Read the model definition and answer for the solid it produces. Units are mm, in the model's axes. Round coordinates to 2 decimals unless told otherwise and drop trailing zeros. Write each loop counter-clockwise with the first axis right and the second up, starting at its lowest first coordinate (ties: lowest second). Pieces come first, ordered by that corner, then holes. Notation, with made-up numbers: (3, -11) - (45, -11) arc R23 ccw to (45, 27) - close; hole circle Ø4 at (56, -14). An arc over 180 degrees is marked (long way). Answer as CSV lines item,"result". Start each with the question number.
1) Find section A-A on x = 0. Determine the outline of the cut face in (y, z) (3 decimals), then the cut area to 3 significant figures.
2) Consider line 1 along Y through (x, z) = (0, -0.4); line 2 along Y through (x, z) = (-0.5, -3); line 3 along X through (y, z) = (15, -2.9) (3 decimals). Determine where each line is inside the solid, lowest interval first.
3) Find section D-D on z = -4. Determine the outline of the cut face in (x, y) (3 decimals), then the cut area to 3 significant figures.
4) Find section C-C on y = 26. Determine the outline of the cut face in (x, z).
5) Each of these flat-tipped pins is pushed along its axis until it touches: pin 1 (2 mm diameter, centred on x = -1.5, y = 15.5, fed in from +Z); pin 2 (2 mm diameter, centred on x = 4.5, y = 54, fed in from +Z); pin 3 (1 mm diameter, centred on y = 36.5, z = -1.5, fed in from -X). Where does it stop, or does it pass through?
6) Find section B-B on y = 45. Determine the outline of the cut face in (x, z) (3 decimals).
from build123d import *

# Parameters (mm, degrees)
BOSS_EXTRUDE1_DEPTH                       = 60
TAPPED_HOLE_FOR_M2_5X0_45_HELICOIL1_D     = 2.55
TAPPED_HOLE_FOR_M2_5X0_45_HELICOIL1_DEPTH = 4
TAPPED_HOLE_FOR_M2_5X0_45_HELICOIL1_TIP   = 0.766097289
F_2_0MM_DOWEL_HOLE1_D                     = 2
F_2_0MM_DOWEL_HOLE1_DEPTH                 = 6.45
F_2_0MM_DOWEL_HOLE1_TIP                   = 0.600860619


with BuildPart() as part:
    # Sketch1 → Boss-Extrude1 (new body)
    with BuildSketch(Plane(origin=(0, 0, 0), x_dir=(1, 0, 0), z_dir=(0, 1, 0))):
        with BuildLine():
            Line((-0.716915426, 0), (0.716915426, 0))
            ThreePointArc((0.716915426, 0), (3.210792252, 3.53742677), (7, 5.629008568))
            Line((7, 5.629008568), (7, 6))
            Line((7, 6), (-7, 6))
            Line((-7, 6), (-7, 5.629008568))
            ThreePointArc((-7, 5.629008568), (-3.210792252, 3.53742677), (-0.716915426, 0))
        make_face()
    extrude(amount=BOSS_EXTRUDE1_DEPTH)

    # Tapped Hole for M2.5x0.45 Helicoil1
    with Locations(Plane(origin=(0, 45, -6), x_dir=(-1, 0, 0), z_dir=(0, 0, -1))):
        with Locations((0, 0), (0, -30)):
            Hole(TAPPED_HOLE_FOR_M2_5X0_45_HELICOIL1_D / 2, depth=TAPPED_HOLE_FOR_M2_5X0_45_HELICOIL1_DEPTH)
            with Locations((0, 0, -(TAPPED_HOLE_FOR_M2_5X0_45_HELICOIL1_DEPTH + TAPPED_HOLE_FOR_M2_5X0_45_HELICOIL1_TIP / 2))):  # 118° drill point
                Cone(0, TAPPED_HOLE_FOR_M2_5X0_45_HELICOIL1_D / 2, TAPPED_HOLE_FOR_M2_5X0_45_HELICOIL1_TIP, mode=Mode.SUBTRACT)

    # Ø2.0mm Dowel Hole1
    with Locations(Plane(origin=(0, 45, -6), x_dir=(-1, 0, 0), z_dir=(0, 0, -1))):
        with Locations((0, 0), (0, -30)):
            Hole(F_2_0MM_DOWEL_HOLE1_D / 2, depth=F_2_0MM_DOWEL_HOLE1_DEPTH)
            with Locations((0, 0, -(F_2_0MM_DOWEL_HOLE1_DEPTH + F_2_0MM_DOWEL_HOLE1_TIP / 2))):  # 118° drill point
                Cone(0, F_2_0MM_DOWEL_HOLE1_D / 2, F_2_0MM_DOWEL_HOLE1_TIP, mode=Mode.SUBTRACT)


solid = part.part
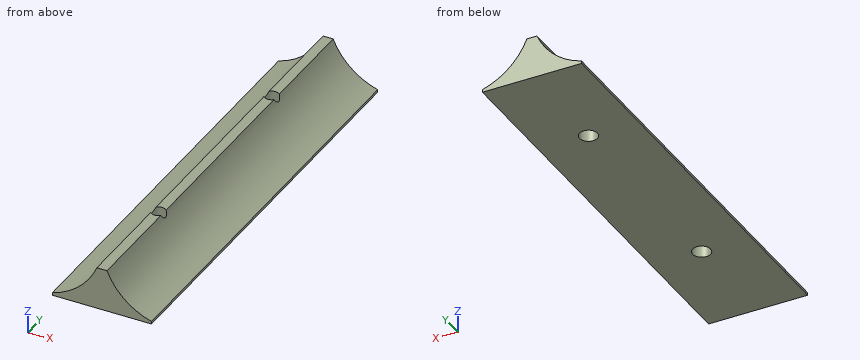
Check values:
1,outline,"(0, -6) - (13.725, -6) - (13.725, -2) - (14, -1.835) - (14, 0) - (0, 0) - close; (16, -1.835) - (16.275, -2) - (16.275, -6) - (43.725, -6) - (43.725, -2) - (44, -1.835) - (44, 0) - (16, 0) - close; (46, -1.835) - (46.275, -2) - (46.275, -6) - (60, -6) - (60, 0) - (46, 0) - close"
1,area,"332 mm^2"
2,line 1,"y = 0 to 14, 16 to 44, 46 to 60"
2,line 2,"y = 0 to 13.83, 16.17 to 43.83, 46.17 to 60"
2,line 3,"x = -2.563 to -1.275, 1.275 to 2.563"
3,outline,"(-3.768, 0) - (3.768, 0) - (3.768, 60) - (-3.768, 60) - close; hole circle Ø2.55 at (0, 15); hole circle Ø2.55 at (0, 45)"
3,area,"442 mm^2"
4,outline,"(-7, -6) - (7, -6) - (7, -5.63) arc R9.65 cw to (0.72, 0) - (-0.72, 0) arc R9.65 cw to (-7, -5.63) - close"
5,pin 1,"stops at z = 0"
5,pin 2,"stops at z = -3.79"
5,pin 3,"stops at x = -1.83"
6,outline,"(-7, -6) - (-1.275, -6) - (-1.275, -2) - (-1, -1.835) - (-1, -0.628) arc R9.65 cw to (-7, -5.629) - close; (1, -1.835) - (1.275, -2) - (1.275, -6) - (7, -6) - (7, -5.629) arc R9.65 cw to (1, -0.628) - close"
